Source: CAD feature listing. Evaluate the final solid. Frame: model axes, mm. A direction names the side the tool comes from. Round coordinates to 2 decimals unless told otherwise and drop trailing zeros. Write each loop counter-clockwise with the first axis right and the second up, starting at its lowest first coordinate (ties: lowest second). Pieces come first, ordered by that corner, then holes. Notation, with made-up numbers: (57, 41) - (114, 41) arc R25 ccw to (114, 64) - close; hole circle Ø1 at (58.25, 38.25). An arc over 180 degrees is marked (long way). Write item = value, one per line. Start each with the question number.
```python
from build123d import *

# Parameters (mm, degrees)
F0_W     = 25.4
F0_H     = 7.9
F1_DEPTH = 12.7
F2_SIZE  = 5.08
F3_W     = 9.652
F3_H     = 7.9
F4_DEPTH = 10.16


with BuildPart() as f1:
    # F0 (on Top) → F1 (new body)
    with BuildSketch(Plane.XY):
        Rectangle(F0_W, F0_H)
    extrude(amount=F1_DEPTH)

    # F2
    f2_edges = [f1.edges().sort_by_distance(p)[0] for p in [
        (12.7, 0, 12.7),
        (-12.7, 0, 12.7),
    ]]
    chamfer(f2_edges, length=F2_SIZE)

    # F3 (on face) → F4 (cut)
    with BuildSketch(Plane.XY.offset(12.7)):
        Rectangle(F3_W, F3_H)
    extrude(amount=-F4_DEPTH, mode=Mode.SUBTRACT)


solid = f1.part
```
(1) Section D-D (x = 4). Return the cut outline in (y, z).
(2) Section A-A (z = 11). Return the cut outline in (x, y).
(3) Pull-direction query (X, two-part tool) for faces 3 (the flat face through (-4.826, 0, 8)), 4 (the flat face through (-12.7, 0, 4)), 5 (the flat face through (12.7, 0, 4)); classes: +X half, -X half, draft (parallel to the pull), parting line (faces both ways), or undercut.
(4) Section C-C (z = 9). Return the cut outline in (x, y), plus the area to 3 significant figures.
(5) Contact query for flat-ended pins moving along their axis: P1, Ø1, axis at x = -2.5, y = -2.5, coming from the +Z side; P2, Ø4, axis at y = -2.5, z = 10, coming from the +X side. Output: stop coordinate, or through.
(6) Section B-B (y = 1.5). Return the cut outline in (x, z), plus the area to 3 significant figures.
(7) Ray query, L1, parallel to X at y = 0.25, z = 3; L2, parallel to Z at x = 1.25, y = 1.25; L3, parallel to X at y = 3, z = 12.25. Return the intervals inside material, ascending. Write a range as from..to.
(8) Reachability of faces 1 (the flat face through (0, -3.95, 2)), 2 (the flat face through (0, 0, 2.54)) from +Z, -Z, +X, -X, +Y, -Y: full face, straight path, thin tool, end or side. Return the list, or none.
Solution:
q1.outline = (-3.95, 0) - (3.95, 0) - (3.95, 2.54) - (-3.95, 2.54) - close
q2.outline = (-9.32, -3.95) - (-4.83, -3.95) - (-4.83, 3.95) - (-9.32, 3.95) - close; (4.83, -3.95) - (9.32, -3.95) - (9.32, 3.95) - (4.83, 3.95) - close
q3.face_3 = undercut
q3.face_4 = -X half
q3.face_5 = +X half
q4.outline = (-11.32, -3.95) - (-4.83, -3.95) - (-4.83, 3.95) - (-11.32, 3.95) - close; (4.83, -3.95) - (11.32, -3.95) - (11.32, 3.95) - (4.83, 3.95) - close
q4.area = 103 mm^2
q5.P1 = 2.54
q5.P2 = 12.32
q6.outline = (-12.7, 0) - (12.7, 0) - (12.7, 7.62) - (7.62, 12.7) - (4.83, 12.7) - (4.83, 2.54) - (-4.83, 2.54) - (-4.83, 12.7) - (-7.62, 12.7) - (-12.7, 7.62) - close
q6.area = 199 mm^2
q7.L1 = -12.7..-4.83, 4.83..12.7
q7.L2 = 0..2.54
q7.L3 = -8.07..-4.83, 4.83..8.07
q8.face_1 = +Z, -Z, +X, -X, -Y
q8.face_2 = +Z, +Y, -Y
